CAD build for the part. Positions are in the model's coordinates, mm. A direction names the side the tool comes from. Coordinates: 2 decimals unless noted, no trailing zeros. Loops run counter-clockwise (first coordinate to the right, second up) from the corner with the lowest first, then second, coordinate; pieces in that order, holes last. Notation, with made-up numbers: (30.5, 29) - (38.5, 29) arc R23 ccw to (38.5, 57) - close; hole circle Ø9 at (-37, 18). An arc over 180 degrees is marked (long way). Put each result on its own line as item: value.
```python
from build123d import *

# Parameters (mm, degrees)
F0_W      = 40
F0_H      = 140
F1_DEPTH  = 5
F2_R      = 19.99999
F3_R      = 4.5
F5_DEPTH  = 5
F6_W      = 12
F6_H      = 12
F7_DEPTH  = 3
F8_R      = 2
F10_DEPTH = 5


# Not quite as in the source:
# - a fillet or chamfer is up to 0.001 mm smaller than in the source, because OpenCascade refuses the exact size
# - a pattern or mirror of a feature is missing from the dataset's text; its kind, count and spacing are read off the source's solid


with BuildPart() as f1:
    # F0 (on Front) → F1 (new body)
    with BuildSketch(Plane.XZ):
        Rectangle(F0_W, F0_H)
    extrude(amount=F1_DEPTH)

    # F2 (radius 20 in the source; OpenCascade refuses exactly that, so slightly less here)
    f2_edges = [f1.edges().sort_by_distance(p)[0] for p in [
        (-20, -2.5, 70),
        (20, -2.5, 70),
        (20, -2.5, -70),
        (-20, -2.5, -70),
    ]]
    fillet(f2_edges, radius=F2_R)

    # F3
    f3_edges = [f1.edges().sort_by_distance(p)[0] for p in [
        (20, -5, 0),
        (0, -5, -70),
        (-14.142139, -5, -64.142139),
        (14.142139, -5, -64.142139),
        (-20, -5, 0),
        (-14.142139, -5, 64.142139),
        (14.142139, -5, 64.142139),
        (0, -5, 70),
    ]]
    fillet(f3_edges, radius=F3_R)

    # F4 (on face) → F5 (join)
    with BuildSketch(Plane(origin=(0, 0, 0), x_dir=(-1, 0, 0), z_dir=(0, 1, 0))):
        with BuildLine():
            ThreePointArc((2.5399159699, 60.1534954225), (2.8826851987, 60.9192617469), (3, 61.75))
            ThreePointArc((3, 61.75), (2.9811636084, 62.0856538989), (2.9248909734, 62.4170927923))
            ThreePointArc((2.9248909734, 62.4170927923), (2.4469615912, 63.48562063), (1.5965045374, 64.2899159951))
            ThreePointArc((1.5965045374, 64.2899159951), (0.5029940174, 64.7075322515), (-0.6670927923, 64.6748909734))
            ThreePointArc((-0.6670927923, 64.6748909734), (-1.7356206048, 64.1969616091), (-2.5399159621, 63.3465045899))
            ThreePointArc((-2.5399159621, 63.3465045899), (-2.9575322502, 62.2529940246), (-2.9248909629, 61.0829071616))
            ThreePointArc((-2.9248909629, 61.0829071616), (-2.4469615928, 60.0143793723), (-1.5965045824, 59.2100840332))
            ThreePointArc((-1.5965045824, 59.2100840332), (-0.5029939825, 58.7924677426), (0.6670929131, 58.8251090541))
            ThreePointArc((0.6670929131, 58.8251090541), (1.7356206613, 59.303038431), (2.5399159699, 60.1534954225))
        make_face()
        with BuildLine():
            ThreePointArc((2.9248909734, 62.4170927923), (2.9811636084, 62.0856538989), (3, 61.75))
            ThreePointArc((3, 61.75), (2.8826851987, 60.9192617469), (2.5399159699, 60.1534954225))
            Line((2.5399159699, 60.1534954225), (3.2012098578, 61.2055632972))
            Line((3.2012098578, 61.2055632972), (2.9248909734, 62.4170927923))
        make_face()
        with BuildLine():
            ThreePointArc((1.5965045374, 64.2899159951), (2.4469615912, 63.48562063), (2.9248909734, 62.4170927923))
            Line((2.9248909734, 62.4170927923), (2.648572083, 63.628622314))
            Line((2.648572083, 63.628622314), (1.5965045374, 64.2899159951))
        make_face()
        with BuildLine():
            Line((1.878622314, 59.101427917), (2.5399159699, 60.1534954225))
            ThreePointArc((2.5399159699, 60.1534954225), (1.7356206613, 59.303038431), (0.6670929131, 58.8251090541))
            Line((0.6670929131, 58.8251090541), (1.878622314, 59.101427917))
        make_face()
        with BuildLine():
            ThreePointArc((-0.6670927923, 64.6748909734), (0.5029940174, 64.7075322515), (1.5965045374, 64.2899159951))
            Line((1.5965045374, 64.2899159951), (0.5444367028, 64.9512098578))
            Line((0.5444367028, 64.9512098578), (-0.6670927923, 64.6748909734))
        make_face()
        with BuildLine():
            Line((-0.5444367028, 58.5487901422), (0.6670929131, 58.8251090541))
            ThreePointArc((0.6670929131, 58.8251090541), (-0.5029939825, 58.7924677426), (-1.5965045824, 59.2100840332))
            Line((-1.5965045824, 59.2100840332), (-0.5444367028, 58.5487901422))
        make_face()
        with BuildLine():
            ThreePointArc((-2.5399159621, 63.3465045899), (-1.7356206048, 64.1969616091), (-0.6670927923, 64.6748909734))
            Line((-0.6670927923, 64.6748909734), (-1.878622314, 64.398572083))
            Line((-1.878622314, 64.398572083), (-2.5399159621, 63.3465045899))
        make_face()
        with BuildLine():
            Line((-2.648572083, 59.871377686), (-1.5965045824, 59.2100840332))
            ThreePointArc((-1.5965045824, 59.2100840332), (-2.4469615928, 60.0143793723), (-2.9248909629, 61.0829071616))
            Line((-2.9248909629, 61.0829071616), (-2.648572083, 59.871377686))
        make_face()
        with BuildLine():
            ThreePointArc((-2.9248909629, 61.0829071616), (-2.9575322502, 62.2529940246), (-2.5399159621, 63.3465045899))
            Line((-2.5399159621, 63.3465045899), (-3.2012098578, 62.2944367028))
            Line((-3.2012098578, 62.2944367028), (-2.9248909629, 61.0829071616))
        make_face()
    f5 = extrude(amount=F5_DEPTH)

    # F5_copies: F5 across plane
    add(f5.mirror(Plane(origin=(0, 0, 0), x_dir=(-1, 0, 0), z_dir=(0, 0, -1))))

    # F6 (on face) → F7 (cut)
    with BuildSketch(Plane(origin=(0, 0, 0), x_dir=(-1, 0, 0), z_dir=(0, 1, 0))):
        with Locations((0, 25.5)):
            Rectangle(F6_W, F6_H)
    f7 = extrude(amount=-F7_DEPTH, mode=Mode.SUBTRACT)

    # F7_copies: F7 across plane
    add(f7.mirror(Plane(origin=(0, 0, 0), x_dir=(-1, 0, 0), z_dir=(0, 0, -1))), mode=Mode.SUBTRACT)

    # F8
    f8_edges = [f1.edges().sort_by_distance(p)[0] for p in [
        (6, -1.5, 31.5),
        (-6, -1.5, 31.5),
        (-6, -1.5, 19.5),
        (6, -1.5, 19.5),
        (6, -1.5, -19.5),
        (-6, -1.5, -19.5),
        (-6, -1.5, -31.5),
        (6, -1.5, -31.5),
    ]]
    fillet(f8_edges, radius=F8_R)

    # F9 (on face) → F10 (join)
    with BuildSketch(Plane(origin=(0, 0, 0), x_dir=(-1, 0, 0), z_dir=(0, 1, 0))):
        with BuildLine():
            ThreePointArc((0, -41), (11.1369318037, -36.3869318037), (15.75, -25.25))
            Line((15.75, -25.25), (15.75, 25.25))
            ThreePointArc((15.75, 25.25), (11.1369318037, 36.3869318037), (0, 41))
            ThreePointArc((0, 41), (-11.1369318037, 36.3869318037), (-15.75, 25.25))
            Line((-15.75, 25.25), (-15.75, -25.25))
            ThreePointArc((-15.75, -25.25), (-11.1369318037, -36.3869318037), (0, -41))
        make_face()
        with BuildLine():
            ThreePointArc((12.75, -25.25), (9.0156114601, -34.2656114601), (0, -38))
            ThreePointArc((0, -38), (-9.0156114601, -34.2656114601), (-12.75, -25.25))
            Line((-12.75, -25.25), (-12.75, 25.25))
            ThreePointArc((-12.75, 25.25), (-9.0156114601, 34.2656114601), (0, 38))
            ThreePointArc((0, 38), (9.0156114601, 34.2656114601), (12.75, 25.25))
            Line((12.75, 25.25), (12.75, -25.25))
        make_face(mode=Mode.SUBTRACT)
    extrude(amount=F10_DEPTH)


solid = f1.part
```
Q1. Tool access for faces 1 (the flat face through (15.75, 2, 0)), 2 (the flat face through (0, -1, 31.5)), 3 (the flat face through (0, 5, 62)): list every direction of +Z, -Z, +X, -X, +Y, -Y with a clear straight run to the whole face (end or side of a thin tool).
Determined:
face 1: +Z, -Z, +X, +Y
face 2: +Y
face 3: +Z, -Z, +X, -X, +Y
Q2. Slice it at B-B, the plane z = -14.5. Give the cut face in (x, y), then the cut area to 3 significant figures.
Determined:
outline: (-20, -0.5) arc R4.5 ccw to (-15.5, -5) - (15.5, -5) arc R4.5 ccw to (20, -0.5) - (20, 0) - (15.75, 0) - (15.75, 5) - (12.75, 5) - (12.75, 0) - (-12.75, 0) - (-12.75, 5) - (-15.75, 5) - (-15.75, 0) - (-20, 0) - close
area: 221 mm2
Q3. Slice it at A-A, the plane y = 3. Give the cut face in (x, z), then the cut area to 3 significant figures.
Determined:
outline: (-15.75, -25.25) arc R15.75 ccw to (15.75, -25.25) - (15.75, 25.25) arc R15.75 ccw to (-15.75, 25.25) - close; (-3.2, -61.21) - (-2.65, -63.63) - (-0.54, -64.95) - (1.88, -64.4) - (3.2, -62.29) - (2.65, -59.87) - (0.54, -58.55) - (-1.88, -59.1) - close; (-3.2, 61.21) - (-1.88, 59.1) - (0.54, 58.55) - (2.65, 59.87) - (3.2, 62.29) - (1.88, 64.4) - (-0.54, 64.95) - (-2.65, 63.63) - close; hole (-12.75, -25.25) arc R12.75 ccw to (12.75, -25.25) - (12.75, 25.25) arc R12.75 ccw to (-12.75, 25.25) - close
area: 631 mm2
Q4. Pin check, flat tips, straight feed: pin 1 Ø3.5 at (x, y) = (-2, -1) entering from +Z; pin 2 Ø10 at (x, z) = (-4, 22.5) entering from +Y; pin 3 Ø2.5 at (y, z) = (-2, 26.5) entering from -X; pin 4 Ø3.5 at (y, z) = (-1, 26) entering from +X. Stop position of each tip, or through.
Determined:
pin 1: z = 70
pin 2: y = 0
pin 3: x = -19.99
pin 4: x = 20
Q5. Mould opens along X. For faces 4 (the flat face through (6, -1, -25)), 5 (the flat face through (0, -5, 1)), 6 (the flat face through (-15.75, 2, 0)) say: +X half, -X half, draft (parallel to the pull), parting line (faces both ways), or undercut.
Determined:
face 4: undercut
face 5: draft
face 6: -X half
Q6. Slice it at C-C, the plane z = -43. Give the cut face in (x, y), then the cut area to 3 significant figures.
Determined:
outline: (-20, -0.5) arc R4.5 ccw to (-15.5, -5) - (15.5, -5) arc R4.5 ccw to (20, -0.5) - (20, 0) - (-20, 0) - close
area: 191 mm2
Q7. Wall check: L1, parallel to X at y = 2, z = 12; L2, parallel to Z at x = 1, y = -2.25; L3, parallel to Z at x = 1.5, y = -0.25. Give the ranges that are in metal, low to high. Write a range as from..to.
Determined:
L1: -15.75..-12.75, 12.75..15.75
L2: -69.62..-31.5, -19.5..19.5, 31.5..69.62
L3: -69.94..-31.5, -19.5..19.5, 31.5..69.94
